Model file for the job. Use its own axes, mm. Face numbers are marked on the shaded views. A direction names the side the tool comes from. Round coordinates to 2 decimals unless told otherwise and drop trailing zeros. Write each loop counter-clockwise with the first axis right and the second up, starting at its lowest first coordinate (ties: lowest second). Pieces come first, ordered by that corner, then holes.
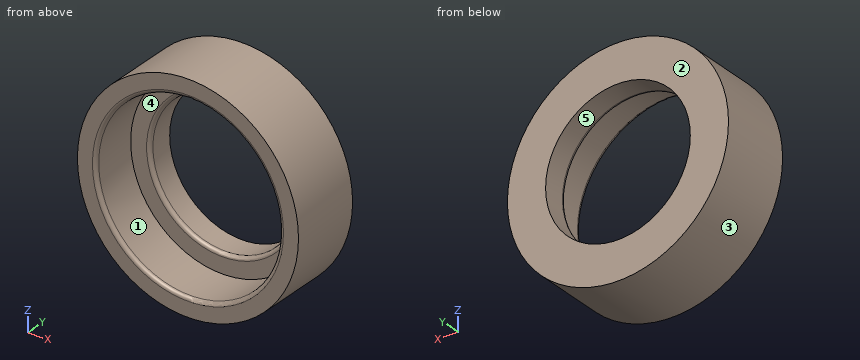
```python
from build123d import *

# Parameters (mm, degrees)
SKETCH1_R           = 30.55
BOSS_EXTRUDE1_DEPTH = 20.32
SKETCH2_R           = 25.404
CUT_EXTRUDE1_DEPTH  = 13
SKETCH3_R           = 20
CUT_EXTRUDE2_DEPTH  = 21.32
FILLET1_R           = 1
FILLET2_R           = 1


with BuildPart() as part:
    # Sketch1 → Boss-Extrude1 (new body)
    with BuildSketch(Plane(origin=(0, 0, 0), x_dir=(1, 0, 0), z_dir=(0, 1, 0))):
        Circle(SKETCH1_R)
    extrude(amount=BOSS_EXTRUDE1_DEPTH)

    # Sketch2 → Cut-Extrude1 (cut)
    with BuildSketch(Plane.XZ):
        Circle(SKETCH2_R)
    extrude(amount=-CUT_EXTRUDE1_DEPTH, mode=Mode.SUBTRACT)

    # Sketch3 → Cut-Extrude2 (cut, through all)
    with BuildSketch(Plane(origin=(0, 20.32, 0), x_dir=(1, 0, 0), z_dir=(0, 1, 0))):
        Circle(SKETCH3_R)
    extrude(amount=-CUT_EXTRUDE2_DEPTH, mode=Mode.SUBTRACT)

    # Fillet1
    fillet1_edges = [part.edges().sort_by_distance(p)[0] for p in [
        (-25.404, 0, 0),
    ]]
    fillet(fillet1_edges, radius=FILLET1_R)

    # Fillet2
    fillet2_edges = [part.edges().sort_by_distance(p)[0] for p in [
        (-20, 13, 0),
    ]]
    fillet(fillet2_edges, radius=FILLET2_R)


solid = part.part
```
1) Wall check: probe 1 along X at (y, z) = (17, 0); probe 2 along X at (y, z) = (9.5, -15). Give the ranges that are in metal, low to high.
2) Pull direction X, two halves, no side cores. Call the marked faces 1, 2 and 3: released by +X, released by -X, zero draft, split by the parting line, or undercut.
3) Cut at A-A on z = 0. List the corners of the cut face in (x, y).
4) Cut at B-B on x = 0. List the corners of the cut face in (y, z), and give its area (3 significant figures).
5) Flat gauge pins, fed straight in: pin 1 Ø6 at (x, y) = (21.5, 16) entering from +Z; pin 2 Ø5 at (x, z) = (12.5, 15) entering from -Y; pin 3 Ø5 at (y, z) = (8.5, -7) entering from -X. Where does each tip first touch, or does it go through?
6) Which spindle directions (+Z, -Z, +X, -X, +Y, -Y) get a long thin tool onto all of the face, cutting with end or side? Do the marked faces 4 and 5. Say none if no direction does.
7) Cut at D-D on y = 9. List the corners of the cut face in (x, z), and give its area (3 significant figures).
8) Cut at C-C on y = 19.25. List the corners of the cut face in (x, z), and give its area (3 significant figures).
Result sheet:
1. probe 1: x = -30.55 to -20, 20 to 30.55
1. probe 2: x = -26.61 to -20.5, 20.5 to 26.61
2. face 1: undercut
2. face 2: zero draft
2. face 3: split by the parting line
3. outline: (-30.55, 0) - (-26.4, 0) arc R1 ccw to (-25.4, 1) - (-25.4, 13) - (-21, 13) arc R1 ccw to (-20, 14) - (-20, 20.32) - (-30.55, 20.32) - close; (20, 14) arc R1 ccw to (21, 13) - (25.4, 13) - (25.4, 1) arc R1 ccw to (26.4, 0) - (30.55, 0) - (30.55, 20.32) - (20, 20.32) - close
4. outline: (0, -30.55) - (20.32, -30.55) - (20.32, -20) - (14, -20) arc R1 ccw to (13, -21) - (13, -25.4) - (1, -25.4) arc R1 ccw to (0, -26.4) - close; (0, 26.4) arc R1 ccw to (1, 25.4) - (13, 25.4) - (13, 21) arc R1 ccw to (14, 20) - (20.32, 20) - (20.32, 30.55) - (0, 30.55) - close
4. area: 287 mm2
5. pin 1: stops at z = 24.31
5. pin 2: stops at y = 13
5. pin 3: stops at x = -30.22
6. face 4: -Y
6. face 5: +Y, -Y
7. outline: circle Ø61.1 at (0, 0); hole circle Ø50.81 at (0, 0)
7. area: 905 mm2
8. outline: circle Ø61.1 at (0, 0); hole circle Ø40 at (0, 0)
8. area: 1,680 mm2
